Geometry: final body of the model. Coordinates: model frame, mm. A direction names the side the tool comes from. Give positions to 0.01 mm unless a question says otherwise; leave off trailing zeros. Answer in a Markdown table with one row per item.
from build123d import *

# Parameters (mm, degrees)
BOSS_EXTRUDE1_DEPTH = 50
CUT_EXTRUDE1_DEPTH  = 50


with BuildPart() as part:
    # Sketch1 → Boss-Extrude1 (new body)
    with BuildSketch(Plane.XY):
        with BuildLine():
            Line((-15, 4), (-13, 4))
            Line((-13, 4), (-13, 8.25))
            Line((-13, 8.25), (-9.664213562, 8.25))
            Line((-9.664213562, 8.25), (-6, 4.585786438))
            Line((-6, 4.585786438), (-6, 0.519615242))
            Line((-6, 0.519615242), (-5.7, 0))
            Line((-5.7, 0), (-5.933012702, -0.403589838))
            ThreePointArc((-5.933012702, -0.403589838), (-6, -0.653589838), (-5.933012702, -0.903589838))
            Line((-5.933012702, -0.903589838), (-5.750976592, -1.218885629))
            Line((-5.750976592, -1.218885629), (-6, -2.5))
            Line((-6, -2.5), (-6, -4.585786438))
            Line((-6, -4.585786438), (-9.664213562, -8.25))
            Line((-9.664213562, -8.25), (-13, -8.25))
            Line((-13, -8.25), (-13, -4))
            Line((-13, -4), (-15, -4))
            Line((-15, -4), (-15, -13))
            ThreePointArc((-15, -13), (-14.414213562, -14.414213562), (-13, -15))
            Line((-13, -15), (-4, -15))
            Line((-4, -15), (-4, -13))
            Line((-4, -13), (-8.25, -13))
            Line((-8.25, -13), (-8.25, -9.664213562))
            Line((-8.25, -9.664213562), (-4.585786438, -6))
            Line((-4.585786438, -6), (-0.519615242, -6))
            Line((-0.519615242, -6), (0, -5.7))
            Line((0, -5.7), (0.403589838, -5.933012702))
            ThreePointArc((0.403589838, -5.933012702), (0.653589838, -6), (0.903589838, -5.933012702))
            Line((0.903589838, -5.933012702), (1.218885629, -5.750976592))
            Line((1.218885629, -5.750976592), (2.5, -6))
            Line((2.5, -6), (4.585786438, -6))
            Line((4.585786438, -6), (8.25, -9.664213562))
            Line((8.25, -9.664213562), (8.25, -13))
            Line((8.25, -13), (4, -13))
            Line((4, -13), (4, -15))
            Line((4, -15), (13, -15))
            ThreePointArc((13, -15), (14.414213562, -14.414213562), (15, -13))
            Line((15, -13), (15, -4))
            Line((15, -4), (13, -4))
            Line((13, -4), (13, -8.25))
            Line((13, -8.25), (9.664213562, -8.25))
            Line((9.664213562, -8.25), (6, -4.585786438))
            Line((6, -4.585786438), (6, -0.519615242))
            Line((6, -0.519615242), (5.7, 0))
            Line((5.7, 0), (5.933012702, 0.403589838))
            ThreePointArc((5.933012702, 0.403589838), (6, 0.653589838), (5.933012702, 0.903589838))
            Line((5.933012702, 0.903589838), (5.750976592, 1.218885629))
            Line((5.750976592, 1.218885629), (6, 2.5))
            Line((6, 2.5), (6, 4.585786438))
            Line((6, 4.585786438), (9.664213562, 8.25))
            Line((9.664213562, 8.25), (13, 8.25))
            Line((13, 8.25), (13, 4))
            Line((13, 4), (15, 4))
            Line((15, 4), (15, 13))
            ThreePointArc((15, 13), (14.414213562, 14.414213562), (13, 15))
            Line((13, 15), (4, 15))
            Line((4, 15), (4, 13))
            Line((4, 13), (8.25, 13))
            Line((8.25, 13), (8.25, 9.664213562))
            Line((8.25, 9.664213562), (4.585786438, 6))
            Line((4.585786438, 6), (0.519615242, 6))
            Line((0.519615242, 6), (0, 5.7))
            Line((0, 5.7), (-0.403589838, 5.933012702))
            ThreePointArc((-0.403589838, 5.933012702), (-0.653589838, 6), (-0.903589838, 5.933012702))
            Line((-0.903589838, 5.933012702), (-1.218885629, 5.750976592))
            Line((-1.218885629, 5.750976592), (-2.5, 6))
            Line((-2.5, 6), (-4.585786438, 6))
            Line((-4.585786438, 6), (-8.25, 9.664213562))
            Line((-8.25, 9.664213562), (-8.25, 13))
            Line((-8.25, 13), (-4, 13))
            Line((-4, 13), (-4, 15))
            Line((-4, 15), (-13, 15))
            ThreePointArc((-13, 15), (-14.414213562, 14.414213562), (-15, 13))
            Line((-15, 13), (-15, 4))
        make_face()
        with BuildLine():
            Line((11.338915743, 9.539070071), (12.361530981, 9.918883282))
            ThreePointArc((12.361530981, 9.918883282), (13.043502884, 13.043502884), (9.918883282, 12.361530981))
            Line((9.918883282, 12.361530981), (9.539070071, 11.338915743))
            ThreePointArc((9.539070071, 11.338915743), (9.861522369, 9.861522369), (11.338915743, 9.539070071))
        make_face(mode=Mode.SUBTRACT)
        with BuildLine():
            Line((9.539070071, -11.338915743), (9.918883282, -12.361530981))
            ThreePointArc((9.918883282, -12.361530981), (13.043502884, -13.043502884), (12.361530981, -9.918883282))
            Line((12.361530981, -9.918883282), (11.338915743, -9.539070071))
            ThreePointArc((11.338915743, -9.539070071), (9.861522369, -9.861522369), (9.539070071, -11.338915743))
        make_face(mode=Mode.SUBTRACT)
        with BuildLine():
            Line((-12.361530981, 9.918883282), (-11.338915743, 9.539070071))
            ThreePointArc((-11.338915743, 9.539070071), (-9.861522369, 9.861522369), (-9.539070071, 11.338915743))
            Line((-9.539070071, 11.338915743), (-9.918883282, 12.361530981))
            ThreePointArc((-9.918883282, 12.361530981), (-13.043502884, 13.043502884), (-12.361530981, 9.918883282))
        make_face(mode=Mode.SUBTRACT)
        with BuildLine():
            Line((-9.918883282, -12.361530981), (-9.539070071, -11.338915743))
            ThreePointArc((-9.539070071, -11.338915743), (-9.861522369, -9.861522369), (-11.338915743, -9.539070071))
            Line((-11.338915743, -9.539070071), (-12.361530981, -9.918883282))
            ThreePointArc((-12.361530981, -9.918883282), (-13.043502884, -13.043502884), (-9.918883282, -12.361530981))
        make_face(mode=Mode.SUBTRACT)
    extrude(amount=-BOSS_EXTRUDE1_DEPTH)

    # Sketch2 → Cut-Extrude1 (cut)
    with BuildSketch(Plane.XY):
        with BuildLine():
            Line((-4.5, -4.8), (-2.644433572, -4.8))
            ThreePointArc((-2.644433572, -4.8), (-2.615679847, -4.79861886), (-2.587190874, -4.794488155))
            Line((-2.587190874, -4.794488155), (-1.742757301, -4.630346896))
            ThreePointArc((-1.742757301, -4.630346896), (-1.568512625, -4.526682207), (-1.5, -4.335858741))
            Line((-1.5, -4.335858741), (-1.5, -3.5))
            ThreePointArc((-1.5, -3.5), (-1.374371466, -3.255879964), (-1.10270272, -3.21621621))
            ThreePointArc((-1.10270272, -3.21621621), (-9e-09, -3.4), (1.102702703, -3.216216216))
            ThreePointArc((1.102702703, -3.216216216), (1.374371458, -3.255879959), (1.5, -3.5))
            Line((1.5, -3.5), (1.5, -4.335858741))
            ThreePointArc((1.5, -4.335858741), (1.568512625, -4.526682207), (1.742757301, -4.630346896))
            Line((1.742757301, -4.630346896), (2.587190874, -4.794488155))
            ThreePointArc((2.587190874, -4.794488155), (2.615679847, -4.79861886), (2.644433572, -4.8))
            Line((2.644433572, -4.8), (4.5, -4.8))
            ThreePointArc((4.5, -4.8), (4.712132034, -4.712132034), (4.8, -4.5))
            Line((4.8, -4.5), (4.8, -2.644433572))
            ThreePointArc((4.8, -2.644433572), (4.79861886, -2.615679847), (4.794488155, -2.587190874))
            Line((4.794488155, -2.587190874), (4.630346896, -1.742757301))
            ThreePointArc((4.630346896, -1.742757301), (4.526682207, -1.568512625), (4.335858741, -1.5))
            Line((4.335858741, -1.5), (3.5, -1.5))
            ThreePointArc((3.5, -1.5), (3.255879964, -1.374371466), (3.21621621, -1.10270272))
            ThreePointArc((3.21621621, -1.10270272), (3.4, -9e-09), (3.216216216, 1.102702703))
            ThreePointArc((3.216216216, 1.102702703), (3.255879959, 1.374371458), (3.5, 1.5))
            Line((3.5, 1.5), (4.335858741, 1.5))
            ThreePointArc((4.335858741, 1.5), (4.526682207, 1.568512625), (4.630346896, 1.742757301))
            Line((4.630346896, 1.742757301), (4.794488155, 2.587190874))
            ThreePointArc((4.794488155, 2.587190874), (4.79861886, 2.615679847), (4.8, 2.644433572))
            Line((4.8, 2.644433572), (4.8, 4.5))
            ThreePointArc((4.8, 4.5), (4.712132034, 4.712132034), (4.5, 4.8))
            Line((4.5, 4.8), (2.644433572, 4.8))
            ThreePointArc((2.644433572, 4.8), (2.615679847, 4.79861886), (2.587190874, 4.794488155))
            Line((2.587190874, 4.794488155), (1.742757301, 4.630346896))
            ThreePointArc((1.742757301, 4.630346896), (1.568512625, 4.526682207), (1.5, 4.335858741))
            Line((1.5, 4.335858741), (1.5, 3.5))
            ThreePointArc((1.5, 3.5), (1.374371466, 3.255879964), (1.10270272, 3.21621621))
            ThreePointArc((1.10270272, 3.21621621), (9e-09, 3.4), (-1.102702703, 3.216216216))
            ThreePointArc((-1.102702703, 3.216216216), (-1.374371458, 3.255879959), (-1.5, 3.5))
            Line((-1.5, 3.5), (-1.5, 4.335858741))
            ThreePointArc((-1.5, 4.335858741), (-1.568512625, 4.526682207), (-1.742757301, 4.630346896))
            Line((-1.742757301, 4.630346896), (-2.587190874, 4.794488155))
            ThreePointArc((-2.587190874, 4.794488155), (-2.615679847, 4.79861886), (-2.644433572, 4.8))
            Line((-2.644433572, 4.8), (-4.5, 4.8))
            ThreePointArc((-4.5, 4.8), (-4.712132034, 4.712132034), (-4.8, 4.5))
            Line((-4.8, 4.5), (-4.8, 2.644433572))
            ThreePointArc((-4.8, 2.644433572), (-4.79861886, 2.615679847), (-4.794488155, 2.587190874))
            Line((-4.794488155, 2.587190874), (-4.630346896, 1.742757301))
            ThreePointArc((-4.630346896, 1.742757301), (-4.526682207, 1.568512625), (-4.335858741, 1.5))
            Line((-4.335858741, 1.5), (-3.5, 1.5))
            ThreePointArc((-3.5, 1.5), (-3.255879964, 1.374371466), (-3.21621621, 1.10270272))
            ThreePointArc((-3.21621621, 1.10270272), (-3.4, 9e-09), (-3.216216216, -1.102702703))
            ThreePointArc((-3.216216216, -1.102702703), (-3.255879959, -1.374371458), (-3.5, -1.5))
            Line((-3.5, -1.5), (-4.335858741, -1.5))
            ThreePointArc((-4.335858741, -1.5), (-4.526682207, -1.568512625), (-4.630346896, -1.742757301))
            Line((-4.630346896, -1.742757301), (-4.794488155, -2.587190874))
            ThreePointArc((-4.794488155, -2.587190874), (-4.79861886, -2.615679847), (-4.8, -2.644433572))
            Line((-4.8, -2.644433572), (-4.8, -4.5))
            ThreePointArc((-4.8, -4.5), (-4.712132034, -4.712132034), (-4.5, -4.8))
        make_face()
    extrude(amount=-CUT_EXTRUDE1_DEPTH, mode=Mode.SUBTRACT)


solid = part.part
Q1. Draft query along Y for faces 1 (the flat face through (1.04, 3.4, -50)), 2 (the flat face through (-8, 15, -25)), 3 (the flat face through (8, -15, -25)), 4 (the flat face through (-7.806, -6.392, -24.65)). Return one class per face: pulls with the +Y half, pulls with the -Y half, needs draft (parallel to the pull), parting line crosses it, or undercut.
Check values:
| item | result |
|---|---|
| face 1 | needs draft |
| face 2 | pulls with the +Y half |
| face 3 | pulls with the -Y half |
| face 4 | undercut |
Q2. Material intervals for line 1 along Y through (x, z) = (11.7, -30.5); line 2 along X through (y, z) = (3.5, -44.5), sorted ascending.
Check values:
| item | result |
|---|---|
| line 1 | -15 to -13.6, -9.67 to -8.25, 8.25 to 9.67, 13.6 to 15 |
| line 2 | -6 to -4.8, -1.5 to 1.5, 4.8 to 6 |
Q3. Cut plane A-A (z = -22.5). Give the number of separate pieces and of enclosed holes in the cut face, and give its area (3 significant figures).
Check values:
| item | result |
|---|---|
| separate pieces | 1 |
| enclosed holes | 5 |
| area | 297 mm² |
Q4. First-contact query: pin 1 (1.6 mm diameter, centred on y = -14, z = -24.5, fed in from +X); pin 2 (1 mm diameter, centred on y = 1.5, z = -10, fed in from -X); pin 3 (6 mm diameter, centred on x = 11.7, y = 11.7, fed in from -Z). Flat tips, straight axial feed; report the tip coordinate or a pass-through.
Check values:
| item | result |
|---|---|
| pin 1 | x = 14.99 |
| pin 2 | x = -6 |
| pin 3 | z = -50 |
Q5. Reachability of faces 5 (the flat face through (-4, 4.8, -25)), 6 (the flat face through (-1.85, 5.874, -24.65)) from +Z, -Z, +X, -X, +Y, -Y: full face, straight path, thin tool, end or side. Return the list, or none.
Check values:
| item | result |
|---|---|
| face 5 | +Z, -Z |
| face 6 | +Z, -Z, +Y |
